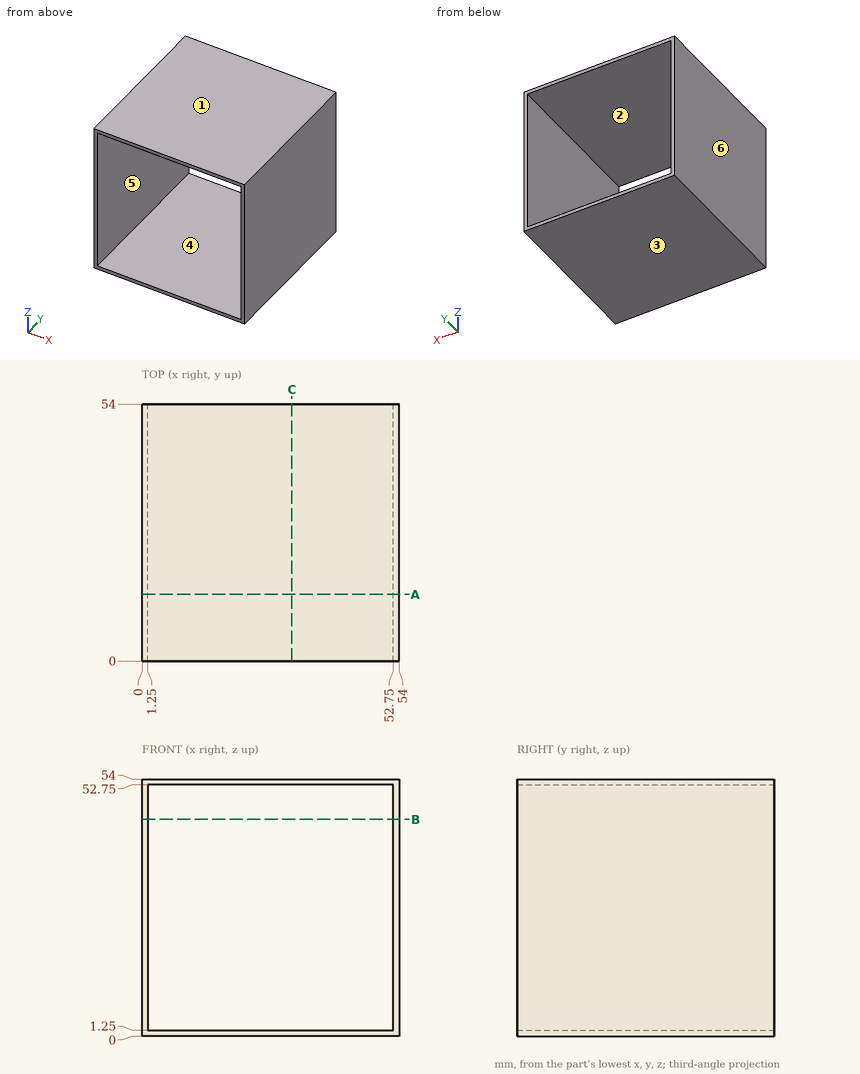
The figure shows three views and two pictorial views of one solid part (mm, origin at its lowest corner). Answer the questions. A direction names the side the tool comes from. Round coordinates to 2 decimals unless told otherwise and drop trailing zeros. Write each loop counter-clockwise with the first axis right and the second up, starting at its lowest first coordinate (ties: lowest second). Pieces come first, ordered by that corner, then holes. Notation, with made-up numbers: (59, 50) -> (100, 50) arc R11 ccw to (100, 68) -> close; hole circle Ø10 at (63.5, -38.75). An arc over 180 degrees is marked (long way). Answer as a JSON object with one key per item and string values. Group by question number.
Q1. Which of the six approach directions +Z, -Z, +X, -X, +Y, -Y give full straight-line access (tool end or side, diameter ignored) to the marked faces 1 and 2?
Q2. Determine the mould class of the marked faces 3, 4, 5 and 6 for opening direction X: pulls with the +X half, pulls with the -X half, needs draft (parallel to the pull), parting line crosses it, or undercut.
Q3. A straight line is drawn through the part: line 1 along Z through (x, y) = (24.5, 3). Find the intervals that lie inside material, in ascending order.
Q4. This flat-tipped pin is pushed along its axis until it touches: pin 1 Ø15.5 at (y, z) = (14, 29) entering from -X. Where does it stop, or does it pass through?
Q5. Section A-A (y = 14) is taken. Write down the section's boundary in (x, z).
Q6. Section B-B (z = 45.5) is taken. Write down the section's boundary in (x, y), plus the area to 3 significant figures.
Q7. Section C-C (x = 31.5) is taken. Write down the section's boundary in (y, z).
Check values:
{
 "1": {"face 1": "+Z, +X, -X, +Y, -Y", "face 2": "+Y, -Y"},
 "2": {"face 3": "needs draft", "face 4": "undercut", "face 5": "undercut", "face 6": "pulls with the -X half"},
 "3": {"line 1": "0 to 1.25, 52.75 to 54"},
 "4": {"pin 1": "x = 0"},
 "5": {"outline": "(0, 0) -> (54, 0) -> (54, 54) -> (0, 54) -> close; hole (1.25, 1.25) -> (52.75, 1.25) -> (52.75, 52.75) -> (1.25, 52.75) -> close"},
 "6": {"outline": "(0, 0) -> (1.25, 0) -> (1.25, 54) -> (0, 54) -> close; (52.75, 0) -> (54, 0) -> (54, 54) -> (52.75, 54) -> close", "area": "135 mm^2"},
 "7": {"outline": "(0, 0) -> (54, 0) -> (54, 1.25) -> (0, 1.25) -> close; (0, 52.75) -> (54, 52.75) -> (54, 54) -> (0, 54) -> close"}
}
